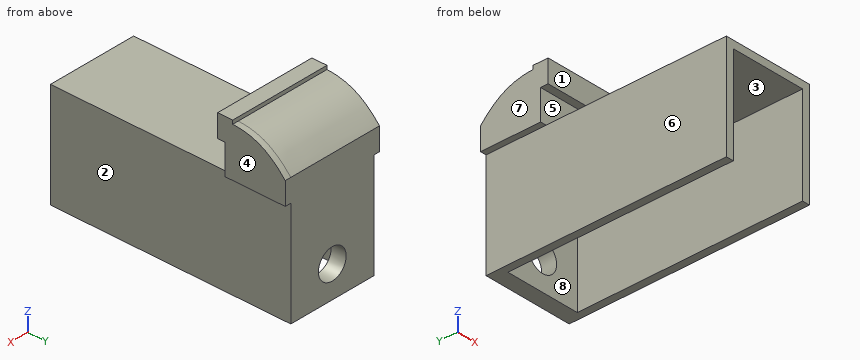
Autodesk Fusion 360 part; units mm, degrees
sketch "Sketch2" plane through (0, 0, 0) normal (0, 1, 0) x (1, 0, 0)
  line L0 (38.1, -44.45) -> (-38.1, -44.45)
  line L1 (-38.1, -44.45) -> (-38.1, 44.45)
  line L2 (-38.1, 44.45) -> (38.1, 44.45)
  line L3 (38.1, 44.45) -> (38.1, -44.45)
  line L4 (38.1, -44.45) -> (-38.1, 44.45) construction
  line L5 (-38.1, -44.45) -> (38.1, 44.45) construction
  dimension "d3" = 76.2
  dimension "d4" = 88.9
extrude "Extrude1" add sketch "Sketch2" along normal blind 203.2
sketch "Sketch3" plane through (0, 0, 0) normal (0, -1, 0) x (1, 0, 0)
  line L0 (-38.1, -44.45) -> (38.1, -44.45)
  line L1 (38.1, -44.45) -> (38.1, 44.45)
  line L2 (38.1, 44.45) -> (-38.1, 44.45)
  line L3 (-38.1, 44.45) -> (-38.1, -44.45)
  line L4 (-31.75, -44.45) -> (31.75, -44.45)
  line L5 (31.75, -44.45) -> (31.75, 38.1)
  line L6 (31.75, 38.1) -> (-31.75, 38.1)
  line L7 (-31.75, 38.1) -> (-31.75, -44.45)
  dimension "d7" = 63.5
  dimension "d8" = 6.35
  dimension "d9" = 6.35
extrude "Extrude2" cut sketch "Sketch3" against normal blind 190.5 contours L0 L4 L5 L6 L7
sketch "Sketch4" plane through (38.1, 0, 0) normal (1, 0, 0) x (0, 1, 0)
  line L0 (0, 44.45) -> (0, -44.45)
  line L1 (0, -44.45) -> (203.2, -44.45)
  line L2 (203.2, -44.45) -> (203.2, 44.45)
  line L3 (203.2, 44.45) -> (0, 44.45)
  line L4 (152.4, 63.4925) -> (203.2, 63.4925)
  line L5 (152.4, 63.4925) -> (152.4, 69.8425)
  line L6 (152.4, 69.8425) -> (158.75, 69.8425)
  line L7 (158.75, 69.8425) -> (158.75, 85.7937)
  line L8 (152.4, 63.4925) -> (152.4, 44.45)
  line L9 (203.2, 63.4925) -> (203.2, 44.45)
  spline S0 degree 5 poles (203.2, 63.4925) (202.0453, 64.8323) (199.6635, 67.4597) (195.8735, 71.2447) (190.3554, 75.9576) (182.304, 81.0202) (174.3584, 83.9897) (167.1278, 85.3037) (161.6519, 85.7089) (158.75, 85.7937) knots 0 0 0 0 0 0 0.2 0.4 0.6 0.8 1 1 1 1 1 1
  line L10 (165.8196, 85.5871) -> (151.6804, 86.0004)
  dimension "d12" = 50.8
  dimension "d13" = 6.35
  dimension "d14" = 15.9512
  dimension "d27" = 19.0426
  dimension "d28" = 6.35
extrude "Extrude3" add sketch "Sketch4" along normal blind 5.08 and the other way blind 81.28 contours L3 L4 L8 L9 | L4 L5 L6 L7 S0
sketch "Sketch5" plane through (0, 158.75, 0) normal (0, -1, 0) x (1, 0, 0)
  line L0 (43.18, 69.8425) -> (43.18, 85.7937)
  line L1 (-43.18, 69.8425) -> (43.18, 69.8425)
  line L2 (-43.18, 85.7937) -> (-43.18, 69.8425)
  line L3 (43.18, 69.8425) -> (-43.18, 69.8425)
  line L4 (-43.18, 69.8425) -> (43.18, 69.8425)
  line L5 (43.18, 69.8425) -> (43.18, 88.8925)
  line L6 (43.18, 88.8925) -> (-43.18, 88.8925)
  line L7 (-43.18, 88.8925) -> (-43.18, 69.8425)
  line L8 (43.18, 85.7937) -> (-43.18, 85.7937)
  dimension "d26" = 19.05
extrude "Extrude4" add sketch "Sketch5" along normal blind 12.7
sketch "Sketch6" plane through (0, 203.2, 0) normal (0, 1, 0) x (-1, 0, 0)
  line L0 (-38.1, -44.45) -> (38.1, -44.45)
  line L1 (38.1, -44.45) -> (38.1, 44.45)
  line L2 (38.1, 44.45) -> (43.18, 44.45)
  line L3 (-43.18, 63.4925) -> (-43.18, 44.45)
  line L4 (43.18, 44.45) -> (43.18, 63.4925)
  line L5 (-38.1, 44.45) -> (-38.1, -44.45)
  circle A0 centre (-0.0873, -17.907) radius 12.7
  line L6 (-0.0873, 10.16) -> (-0.0873, -53.34) construction
  line L7 (43.18, 63.4925) -> (-43.18, 63.4925)
  line L8 (-43.18, 44.45) -> (-38.1, 44.45)
  dimension "d23" = 25.4
  dimension "d25" = 26.543
extrude "Extrude5" cut sketch "Sketch6" against normal through all contours A0
Source: CAD feature listing. Evaluate the final solid. Frame: model axes, mm. Face numbers are marked on the shaded views. A direction names the side the tool comes from. Give positions to 0.01 mm unless a question says otherwise; leave off trailing zeros. Write each loop counter-clockwise with the first axis right and the second up, starting at its lowest first coordinate (ties: lowest second). Pieces come first, ordered by that corner, then holes. Notation, with made-up numbers: M -20.5,-12.75 L 35.5,-12.75 A9 cw 35.5,-1.75 Z; hole C 12.25,52.25 d8. An arc over 180 degrees is marked long. Return JSON: item names as keys, results as strings. Group by question number.
1) Cut plane D-D, the plane z = 53. Output: boundary loops of the cut face in (x, y).
2) Cut plane A-A, the plane z = -9.5. Output: boundary loops of the cut face in (x, y), plus the area to 3 significant figures.
3) Pin query (flat end, axial travel): P1, Ø12, axis at x = -0.5, z = -2, coming from the -Y side; P2, Ø2, axis at y = 91, z = 40, coming from the +X side; P3, Ø6, axis at y = 115, z = 11, coming from the -X side. Return the tip coordinate at first contact, or that it passes through.
4) Cut plane B-B, the plane y = 90. Output: boundary loops of the cut face in (x, z), plus the area to 3 significant figures.
5) Material intervals for line 1 along X through (y, z) = (188, -22.5); line 2 along Z through (x, y) = (11.5, 150); line 3 along Z through (x, y) = (31, 71), sorted ascending. Write a range as [from, to].
6) Pull-direction query (X, two-part tool) for the marked faces 1, 2 and 3; classes: pulls with the +X half, pulls with the -X half, needs draft (parallel to the pull), parting line crosses it, or undercut.
7) Set-up query: the marked faces 4, 5, 6, 7 and 8. Return all of +Z, -Z, +X, -X, +Y, -Y with unobstructed straight access to the full face (end or side cutting, diameter ignored); none if empty.
8) Cut plane C-C, the plane z = 11. Output: boundary loops of the cut face in (x, y).
Recorded:
{
 "1": {"outline": "M -43.18,152.4 L 43.18,152.4 L 43.18,203.2 L -43.18,203.2 Z"},
 "2": {"outline": "M -38.1,0 L -31.75,0 L -31.75,190.5 L -9.43,190.5 L -9.43,203.2 L -38.1,203.2 Z; M 9.61,190.5 L 31.75,190.5 L 31.75,0 L 38.1,0 L 38.1,203.2 L 9.61,203.2 Z", "area": "3,150 mm²"},
 "3": {"P1": "stops at y = 190.5", "P2": "stops at x = 38.1", "P3": "stops at x = -38.1"},
 "4": {"outline": "M -38.1,-44.45 L -31.75,-44.45 L -31.75,38.1 L 31.75,38.1 L 31.75,-44.45 L 38.1,-44.45 L 38.1,44.45 L -38.1,44.45 Z", "area": "1,530 mm²"},
 "5": {"line 1": "x = [-38.1, -31.75], [31.75, 38.1]", "line 2": "z = [38.1, 44.45], [69.84, 88.89]", "line 3": "z = [38.1, 44.45]"},
 "6": {"face 1": "needs draft", "face 2": "pulls with the +X half", "face 3": "undercut"},
 "7": {"face 4": "+Z, -Z, +X, +Y, -Y", "face 5": "+X, -X, -Y", "face 6": "-Z, -X, +Y, -Y", "face 7": "+Z, -Z, -X, +Y, -Y", "face 8": "-Z, -Y"},
 "8": {"outline": "M -38.1,0 L -31.75,0 L -31.75,190.5 L 31.75,190.5 L 31.75,0 L 38.1,0 L 38.1,203.2 L -38.1,203.2 Z"}
}
